Build history of the part. All positions in model axes, mm. Face numbers are marked on the shaded views. A direction names the side the tool comes from. Coordinates: 2 decimals unless noted, no trailing zeros. Order: outer loops, then holes, each group sorted by start corner. A loop starts at its lowest first (then second) coordinate and runs counter-clockwise, first axis right, second up. Notation, with made-up numbers: (84, -29) - (102, -29) arc R27 ccw to (102, -8) - close; hole circle Ø10 at (31, 14). An arc over 180 degrees is marked (long way). One line per item, written item: value.
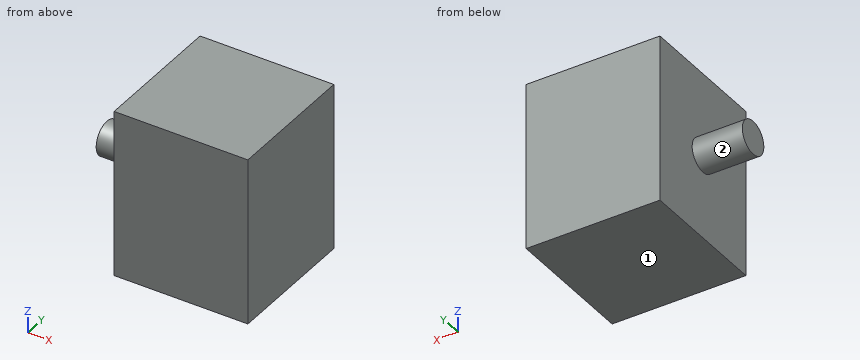
from build123d import *

# Parameters (mm, degrees)
SKETCH2_W           = 16
SKETCH2_H           = 16
BOSS_EXTRUDE1_DEPTH = 20
SKETCH3_R           = 2
BOSS_EXTRUDE2_DEPTH = 6


with BuildPart() as part:
    # Sketch2 → Boss-Extrude1 (new body)
    with BuildSketch(Plane.XY):
        Rectangle(SKETCH2_W, SKETCH2_H)
    extrude(amount=BOSS_EXTRUDE1_DEPTH)

    # Sketch3 → Boss-Extrude2 (add)
    with BuildSketch(Plane.ZY.offset(8)):
        with Locations((10, 0)):
            Circle(SKETCH3_R)
    extrude(amount=BOSS_EXTRUDE2_DEPTH)


solid = part.part
1. 3-axis set-ups, long thin cutter, end or side, ignore diameter. For the marked faces 1 and 2: which of +Z, -Z, +X, -X, +Y, -Y reach the whole face in a straight line?
Values found:
face 1: -Z, +X, -X, +Y, -Y
face 2: -X
2. Band-saw the part on B-B, the plane z = 10. Give the cut face in (x, y).
Values found:
outline: (-14, -2) - (-8, -2) - (-8, -8) - (8, -8) - (8, 8) - (-8, 8) - (-8, 2) - (-14, 2) - close
3. Band-saw the part on C-C, the plane y = 3. Give the cut face in (x, z), and give its area (3 significant figures).
Values found:
outline: (-8, 0) - (8, 0) - (8, 20) - (-8, 20) - close
area: 320 mm2
4. Probe line 1 along X through (y, z) = (3, 18.25); line 2 along Y through (x, z) = (-12, 11.75); line 3 along Z through (x, y) = (-12.5, 1.5). List the from-to ranges inside material, lowest first.
Values found:
line 1: x = -8 to 8
line 2: y = -0.97 to 0.97
line 3: z = 8.68 to 11.32
5. Band-saw the part on A-A, the plane y = 0. Give the cut face in (x, z), and give its area (3 significant figures).
Values found:
outline: (-14, 8) - (-8, 8) - (-8, 0) - (8, 0) - (8, 20) - (-8, 20) - (-8, 12) - (-14, 12) - close
area: 344 mm2
6. Band-saw the part on D-D, the plane z = 17. Give the cut face in (x, y), and give its area (3 significant figures).
Values found:
outline: (-8, -8) - (8, -8) - (8, 8) - (-8, 8) - close
area: 256 mm2
